Check sheet for the drawn part. Datum: minimum x, y, z corner. Units: mm. A direction names the side the tool comes from. Coordinates: 2 decimals unless noted, no trailing zeros. Write each loop counter-clockwise with the first axis right and the second up, starting at its lowest first coordinate (ties: lowest second). Pieces come first, ordered by that corner, then holes. Notation, with made-up numbers: M 80.5,9 L 123.5,9 A6 ccw 123.5,16 Z; hole C 31.25,24.5 d8. An arc over 180 degrees is marked long. Answer as CSV lines item,"result".
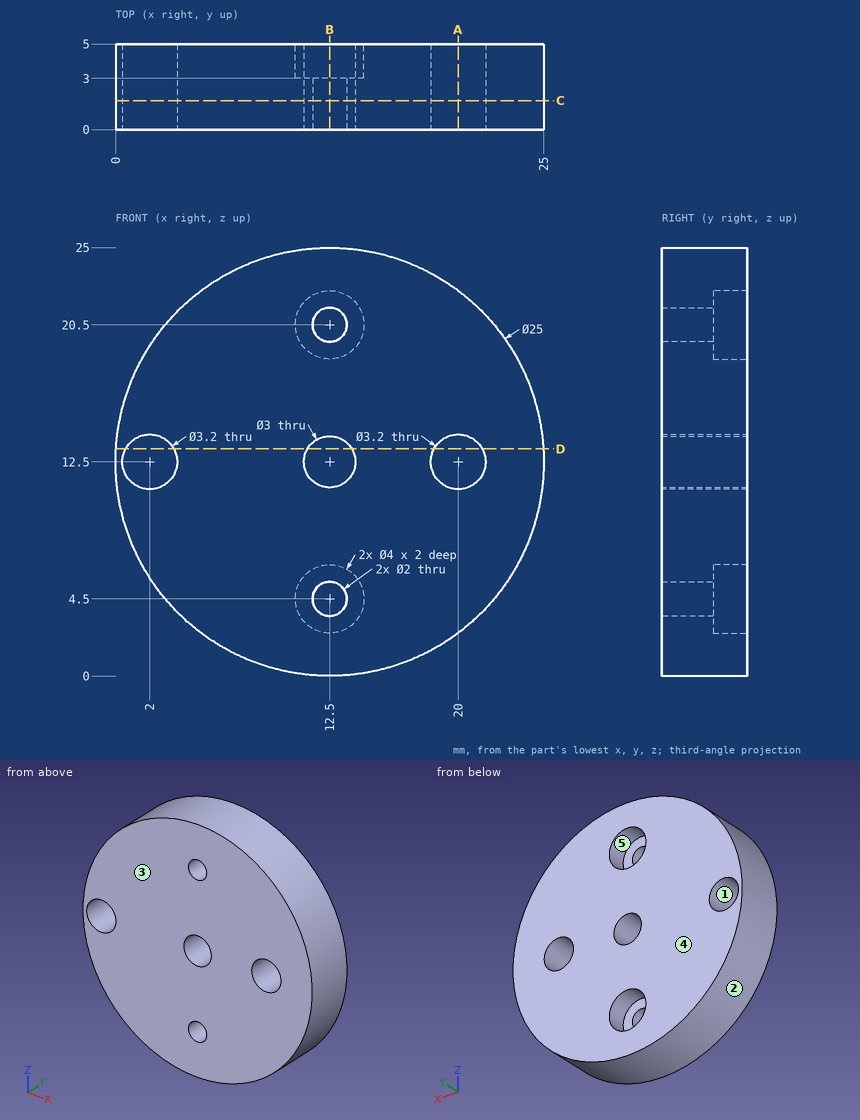
1) Tool access check on the marked faces 4 and 5. Record the directions out of +Z, -Z, +X, -X, +Y, -Y that give a thin tool (end or side, any length) a straight path to the whole face; none if there is none.
Answer key:
face 4,"+Z, -Z, +X, -X, +Y"
face 5,"+Y"
2) Section check D-D, the plane z = 13.25. Record the boundary of the cut face in (x, y).
Answer key:
outline,"M 0.02,0 L 0.59,0 L 0.59,5 L 0.02,5 Z; M 3.41,0 L 11.2,0 L 11.2,5 L 3.41,5 Z; M 13.8,0 L 18.59,0 L 18.59,5 L 13.8,5 Z; M 21.41,0 L 24.98,0 L 24.98,5 L 21.41,5 Z"
3) Section check C-C, the plane y = 1.7. Record the boundary of the cut face in (x, z).
Answer key:
outline,"C 12.5,12.5 d25; hole C 2,12.5 d3.2; hole C 12.5,12.5 d3; hole C 12.5,4.5 d2; hole C 12.5,20.5 d2; hole C 20,12.5 d3.2"
4) Thickness scan on line 1 along X through (y, z) = (3.65, 12.5); line 2 along X through (y, z) = (1.4, 13.5); line 3 along Z through (x, y) = (14.25, 3.8). Record the ranges inside material, lowest first.
Answer key:
line 1,"x = 0 to 0.4, 3.6 to 11, 14 to 18.4, 21.6 to 25"
line 2,"x = 0.04 to 0.75, 3.25 to 11.38, 13.62 to 18.75, 21.25 to 24.96"
line 3,"z = 0.12 to 3.53, 5.47 to 19.53, 21.47 to 24.88"
5) Mould release check, pull along Z, two halves, no side actions. Record for the marked faces 1, 2 and 3: pulls with the +Z half, pulls with the -Z half, needs draft (parallel to the pull), parting line crosses it, or undercut.
Answer key:
face 1,"undercut"
face 2,"parting line crosses it"
face 3,"needs draft"
6) Depth check by flat-ended pin: P1, Ø3, axis at x = 12.5, z = 20.5, coming from the +Y side; P2, Ø2.5, axis at x = 20, z = 12.5, coming from the -Y side; P3, Ø1, axis at x = 21, y = 3.5, coming from the -Z side. Enter the tip coordinate at first touch or a pass-through.
Answer key:
P1,"stops at y = 3"
P2,"passes through"
P3,"stops at z = 2.9"
7) Section check B-B, the plane x = 12.5. Record the boundary of the cut face in (y, z), plus the area to 3 significant figures.
Answer key:
outline,"M 0,0 L 5,0 L 5,2.5 L 3,2.5 L 3,3.5 L 0,3.5 Z; M 0,5.5 L 3,5.5 L 3,6.5 L 5,6.5 L 5,11 L 0,11 Z; M 0,14 L 5,14 L 5,18.5 L 3,18.5 L 3,19.5 L 0,19.5 Z; M 0,21.5 L 3,21.5 L 3,22.5 L 5,22.5 L 5,25 L 0,25 Z"
area,"82.0 mm2"
8) Section check A-A, the plane x = 20. Record the boundary of the cut face in (y, z).
Answer key:
outline,"M 0,2.5 L 5,2.5 L 5,10.9 L 0,10.9 Z; M 0,14.1 L 5,14.1 L 5,22.5 L 0,22.5 Z"
